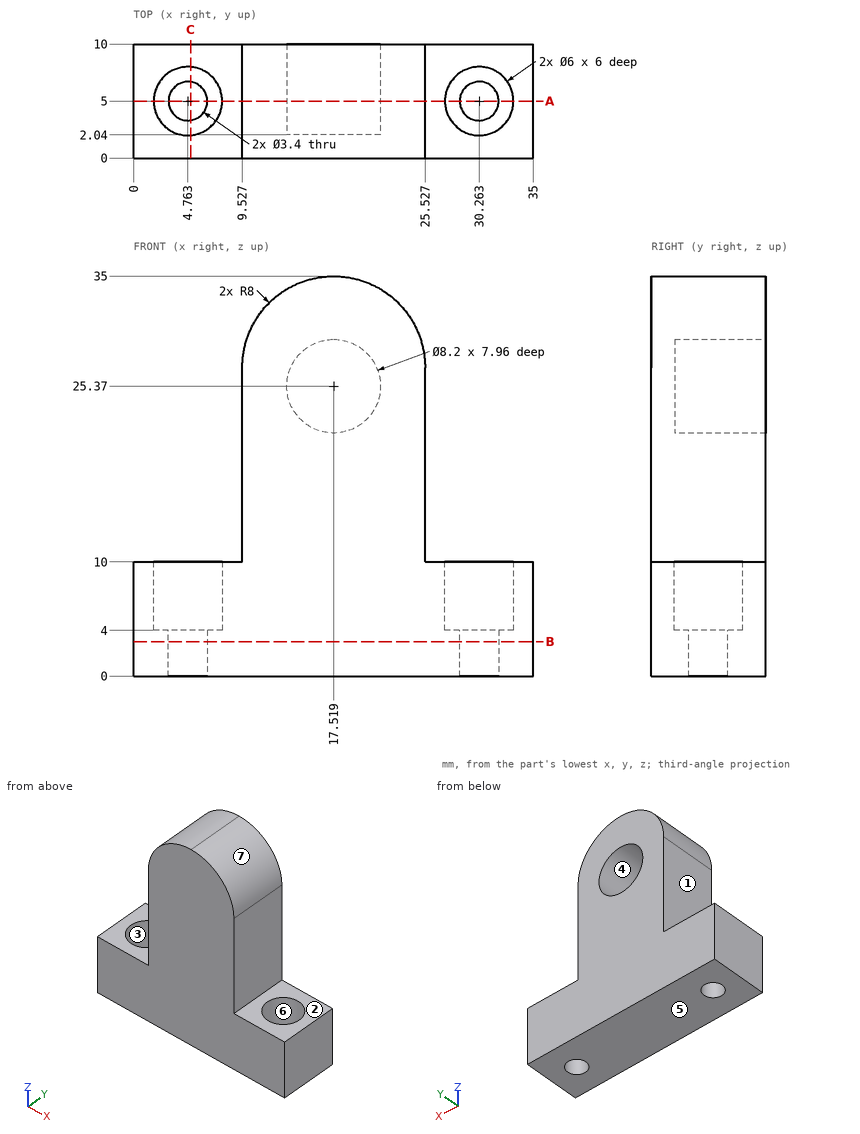
Input: dimensioned drawing with shaded views. Units: mm. Origin: part minimum x, y, z. A direction names the side the tool comes from. Give positions to 0.01 mm unless a question says otherwise; leave off trailing zeros. Loops run counter-clockwise (first coordinate to the right, second up) from the corner with the lowest first, then second, coordinate; pieces in that order, holes last. Notation, with made-up numbers: (51, 16.25) -> (109, 16.25) arc R22 cw to (109, 23.25) -> close; hole circle Ø6 at (-3, -16). An arc over 180 degrees is marked (long way). Use a Markdown table: item, result. Add a question column.
1) Section query B-B, the plane z = 3. Return the cut outline in (x, y), then the cut area to 3 significant figures.
2) Section query A-A, the plane y = 5. Count the separate pieces of the cut face and the enclosed holes in it.
3) Reachability of the marked faces 1, 2, 3 and 4 from +Z, -Z, +X, -X, +Y, -Y: full face, straight path, thin tool, end or side. Return the list, or none.
4) Pull-direction query (X, two-part tool) for the marked faces 5, 6 and 7; classes: +X half, -X half, draft (parallel to the pull), parting line (faces both ways), or undercut.
5) Section query C-C, the plane x = 5. Return the cut outline in (y, z).
6) First-contact query: pin 1 (5 mm diameter, centred on x = 4.76, y = 5, fed in from +Z); pin 2 (2.5 mm diameter, centred on x = 18.5, z = 24.5, fed in from +Y); pin 3 (4 mm diameter, centred on x = 12, y = 6.5, fed in from +Z). Flat tips, straight axial feed; report the tip coordinate or a pass-through.
7) Line query: line 1 along X through (y, z) = (4.75, 2) (1 decimal); line 2 along Z through (x, y) = (6.5, 7.25); line 3 along Z through (x, y) = (22.5, 8) (1 decimal). Output: solid intervals per line, ascending. Write a range as [from, to].
Numbers:
| question | item | result |
|---|---|---|
| 1 | outline | (0, 0) -> (35, 0) -> (35, 10) -> (0, 10) -> close; hole circle Ø3.4 at (4.76, 5); hole circle Ø3.4 at (30.26, 5) |
| 1 | area | 332 mm2 |
| 2 | separate pieces | 3 |
| 2 | enclosed holes | 1 |
| 3 | face 1 | +Z, -X, +Y, -Y |
| 3 | face 2 | +Z, +X, +Y, -Y |
| 3 | face 3 | +Z |
| 3 | face 4 | +Y |
| 4 | face 5 | draft |
| 4 | face 6 | undercut |
| 4 | face 7 | +X half |
| 5 | outline | (0, 0) -> (3.32, 0) -> (3.32, 4) -> (2.01, 4) -> (2.01, 10) -> (0, 10) -> close; (6.68, 0) -> (10, 0) -> (10, 10) -> (7.99, 10) -> (7.99, 4) -> (6.68, 4) -> close |
| 6 | pin 1 | stops at z = 4 |
| 6 | pin 2 | stops at y = 2.04 |
| 6 | pin 3 | stops at z = 34.18 |
| 7 | line 1 | x = [0, 3.1], [6.4, 28.6], [31.9, 35] |
| 7 | line 2 | z = [0, 4] |
| 7 | line 3 | z = [0, 33.3] |
